```python
from build123d import *

# Parameters (mm, degrees)
SKETCH_1_R          = 9.5
EXTRUDE_1_DEPTH     = 3
SKETCH_2_R          = 4
CUT_EXTRUDE_1_DEPTH = 7
SKETCH_3_R          = 7.75
SKETCH_3_R_2        = 5.25
CUT_EXTRUDE_2_DEPTH = 0.5


with BuildPart() as part:
    # 草圖1 → 填料-伸長1 (new body, symmetric)
    with BuildSketch(Plane.XY):
        Circle(SKETCH_1_R)
    extrude(amount=EXTRUDE_1_DEPTH, both=True)

    # 草圖2 → 除料-伸長1 (cut, through all)
    with BuildSketch(Plane.XY.offset(3)):
        Circle(SKETCH_2_R)
    extrude(amount=-CUT_EXTRUDE_1_DEPTH, mode=Mode.SUBTRACT)

    # 草圖3 → 除料-伸長2 (cut)
    with BuildSketch(Plane.XY.offset(3)):
        Circle(SKETCH_3_R)
        Circle(SKETCH_3_R_2, mode=Mode.SUBTRACT)
    cut_extrude_2 = extrude(amount=-CUT_EXTRUDE_2_DEPTH, mode=Mode.SUBTRACT)

    # 鏡射1: 除料-伸長2 across plane
    add(cut_extrude_2.mirror(Plane.XY), mode=Mode.SUBTRACT)


solid = part.part
```
Check sheet for the modelled part. Datum: model origin and axes. Units: mm. A direction names the side the tool comes from. Give positions to 0.01 mm unless a question says otherwise; leave off trailing zeros. Write each loop counter-clockwise with the first axis right and the second up, starting at its lowest first coordinate (ties: lowest second). Pieces come first, ordered by that corner, then holes.
Item 1: Draft check along Y on faces 1 (the face through (-1.009, 7.684, 2.754)), 2 (the face through (-4, -2, -3)), 3 (the face through (4.38, -8.43, 0.04)). Enter one of: released by +Y, released by -Y, zero draft, split by the parting line, or undercut.
Item 2: Cross-section at A-A (y = 0). Enter the section's corners in (x, z).
Item 3: Gauge pin test, flat ends, axial feed: pin 1 (2 mm diameter, centred on x = 7.5, z = -2, fed in from +Y); pin 2 (1 mm diameter, centred on y = -7, z = 0, fed in from +X); pin 3 (3 mm diameter, centred on y = -4.5, z = 1.5, fed in from -X). Record the tip position at first contact, or that the pin passes through.
Item 4: Scan lines: L1, parallel to Y at x = 0, z = 2.6; L2, parallel to X at y = 2.5, z = 2.7; L3, parallel to Y at x = -0.5, z = 0.9. Record each from-to range of solid material in increasing order.
Item 5: Cross-section at C-C (z = -1). Enter the section's corners in (x, y), and give its area (3 significant figures).
Item 6: Access from +Z, -Z, +X, -X, +Y, -Y to the whole of each face (thin tool, end or side, straight path). Record for faces 4 (the face through (-1.8, -5.1, -2.5)), 5 (the face through (-1.8, -5.1, 2.5)), 6 (the face through (-8, 0, 3)).
Item 7: Cross-section at D-D (x = -7). Enter the section's corners in (y, z).
Report:
1. face 1: undercut
1. face 2: zero draft
1. face 3: split by the parting line
2. outline: (-9.5, -3) - (-7.75, -3) - (-7.75, -2.5) - (-5.25, -2.5) - (-5.25, -3) - (-4, -3) - (-4, 3) - (-5.25, 3) - (-5.25, 2.5) - (-7.75, 2.5) - (-7.75, 3) - (-9.5, 3) - close; (4, -3) - (5.25, -3) - (5.25, -2.5) - (7.75, -2.5) - (7.75, -3) - (9.5, -3) - (9.5, 3) - (7.75, 3) - (7.75, 2.5) - (5.25, 2.5) - (5.25, 3) - (4, 3) - close
3. pin 1: stops at y = 6.93
3. pin 2: stops at x = 6.93
3. pin 3: stops at x = -9.01
4. L1: y = -9.5 to -7.75, -5.25 to -4, 4 to 5.25, 7.75 to 9.5
4. L2: x = -9.17 to -7.34, -4.62 to -3.12, 3.12 to 4.62, 7.34 to 9.17
4. L3: y = -9.49 to -3.97, 3.97 to 9.49
5. outline: circle Ø19 at (0, 0); hole circle Ø8 at (0, 0)
5. area: 233 mm2
6. face 4: -Z
6. face 5: +Z
6. face 6: +Z, +X, -X, +Y, -Y
7. outline: (-6.42, -3) - (-3.33, -3) - (-3.33, -2.5) - (3.33, -2.5) - (3.33, -3) - (6.42, -3) - (6.42, 3) - (3.33, 3) - (3.33, 2.5) - (-3.33, 2.5) - (-3.33, 3) - (-6.42, 3) - close
